Here's the drawing with two shaded views (mm, measured from the low corner). I have some questions. Coordinates: 2 decimals unless noted, no trailing zeros. Write each loop counter-clockwise with the first axis right and the second up, starting at its lowest first coordinate (ties: lowest second). Pieces come first, ordered by that corner, then holes.
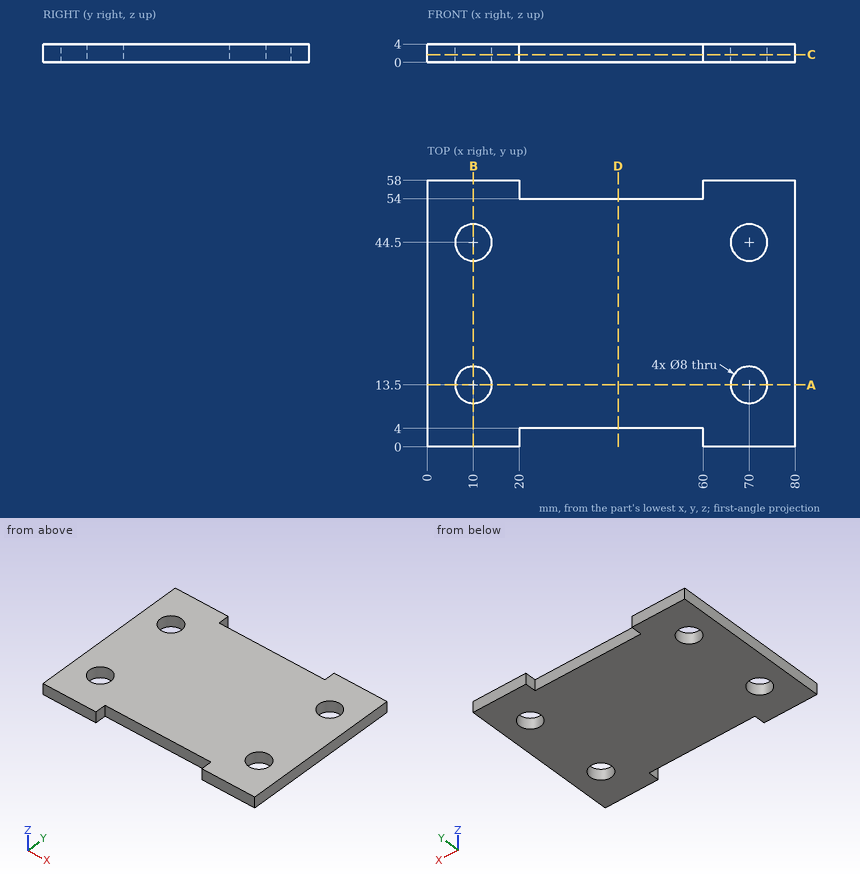
1. For pin 1 (10.5 mm diameter, centred on x = 70, y = 13.5, fed in from +Z); pin 2 (1.5 mm diameter, centred on x = 31.5, z = 2.5, fed in from +Y), each with a flat end and sliding along its axis, tell me the tip position at first contact or that it passes through.
Verdict:
pin 1: stops at z = 4
pin 2: stops at y = 54
2. Please list where these lines run through material, in increasing order: line 1 along Y through (x, z) = (70, 1.2); line 2 along X through (y, z) = (54.5, 0.95); line 3 along Y through (x, z) = (7.5, 3.3).
Verdict:
line 1: y = 0 to 9.5, 17.5 to 40.5, 48.5 to 58
line 2: x = 0 to 20, 60 to 80
line 3: y = 0 to 10.38, 16.62 to 41.38, 47.62 to 58
3. I want a section at A-A on y = 13.5. Please give me the cut outline in (x, z), plus the area to 3 significant figures.
Verdict:
outline: (0, 0) - (6, 0) - (6, 4) - (0, 4) - close; (14, 0) - (66, 0) - (66, 4) - (14, 4) - close; (74, 0) - (80, 0) - (80, 4) - (74, 4) - close
area: 256 mm2
4. I want a section at C-C on z = 1.7. Please give me the cut outline in (x, y).
Verdict:
outline: (0, 0) - (20, 0) - (20, 4) - (60, 4) - (60, 0) - (80, 0) - (80, 58) - (60, 58) - (60, 54) - (20, 54) - (20, 58) - (0, 58) - close; hole circle Ø8 at (10, 13.5); hole circle Ø8 at (10, 44.5); hole circle Ø8 at (70, 13.5); hole circle Ø8 at (70, 44.5)
5. I want a section at D-D on x = 41.5. Please give me the cut outline in (y, z), plus the area to 3 significant figures.
Verdict:
outline: (4, 0) - (54, 0) - (54, 4) - (4, 4) - close
area: 200 mm2
6. I want a section at B-B on x = 10. Please give me the cut outline in (y, z), plus the area to 3 significant figures.
Verdict:
outline: (0, 0) - (9.5, 0) - (9.5, 4) - (0, 4) - close; (17.5, 0) - (40.5, 0) - (40.5, 4) - (17.5, 4) - close; (48.5, 0) - (58, 0) - (58, 4) - (48.5, 4) - close
area: 168 mm2
